Could you check a few things on this model? Use its own coordinates, in mm. A direction names the side the tool comes from. Coordinates: 2 decimals unless noted, no trailing zeros. Order: outer loops, then holes, each group sorted by start corner. A loop starts at its lowest first (then second) coordinate and runs counter-clockwise, first axis right, second up. Notation, with made-up numbers: (83, 18.25) -> (109, 18.25) arc R25 cw to (109, 47.25) -> close; hole circle Ø10 at (73.25, 80). An arc over 180 degrees is marked (long way). Use a Markdown table: item, result. Add a question column.
1) Thinking about a two-plate mould opening in Z: for faces 1 (the flat face through (19, 13, 5.802)), 2 (the flat face through (16.393, 29.272, -7.317)), 3 (the flat face through (17.3, 23.7, -7.1)), which applies, +Z half, -Z half, draft (parallel to the pull), parting line (faces both ways), or undercut?
2) If we section it at C-C (z = 4): Write out the boundary of the cut face in (x, y).
3) If I drill on L1, parallel to Z at x = 12.5, y = 17; L2, parallel to Y at x = 9.5, z = -11.25; L3, parallel to X at y = 15.25, z = -8, over which ranges is the centre line in solid material (lowest first)? Write a range as [from, to].
4) Will these pins go through, and if not, where does the flat tip stop? pin 1 Ø8 at (x, z) = (8, -13) entering from +Y; pin 2 Ø6 at (x, y) = (13.5, 20.5) entering from +Z; pin 3 Ø8 at (y, z) = (21, -3) entering from +X.
5) If we section it at B-B (x = 38): Write out the boundary of the cut face in (y, z).
6) Which directions (+Z, -Z, +X, -X, +Y, -Y) give clear straight access to the entire face, cutting with the end or side of a thin tool? Please do faces 4 (the flat face through (15, 21, -15.698)), 5 (the flat face through (18, 14, -2.957)), 6 (the flat face through (13, 18, -2.948)).
7) If we section it at A-A (z = -8.75): Write out the boundary of the cut face in (x, y), plus the area to 3 significant figures.
```python
from build123d import *

# Parameters (mm, degrees)
ESBO_O1_R                  = 1.5
RESSALTO_EXTRUS_O1_DEPTH   = 12
RESSALTO_EXTRUS_O1_2_DEPTH = 12
ESBO_O1_R_2                = 1.500000005
RESSALTO_EXTRUS_O1_3_DEPTH = 12
RESSALTO_EXTRUS_O1_4_DEPTH = 12
RESSALTO_EXTRUS_O1_5_DEPTH = 12
RESSALTO_EXTRUS_O1_6_DEPTH = 12
ESBO_O1_R_3                = 1.500000003
RESSALTO_EXTRUS_O1_7_DEPTH = 12
RESSALTO_EXTRUS_O1_8_DEPTH = 12
ESBO_O2_W                  = 79.998506149
ESBO_O2_H                  = 25.999999951
RESSALTO_EXTRUS_O2_DEPTH   = 3
ESBO_O3_W                  = 15
ESBO_O3_H                  = 17
RESSALTO_EXTRUS_O3_DEPTH   = 15
CHANFRO1_START             = 28.832866647
CHANFRO1_OUTLINE_W         = 17.320508076
CHANFRO1_OUTLINE_H         = 17
CHANFRO1_DEPTH             = 8.167133353
ESBO_O4_R                  = 7.5
CORTE_EXTRUS_O3_DEPTH      = 2
ESBO_O5_R                  = 3
CORTE_EXTRUS_O4_DEPTH      = 2
ESBO_O6_W                  = 8.5
ESBO_O6_H                  = 8.5
CORTE_EXTRUS_O5_DEPTH      = 9
ESBO_O7_W                  = 8.495190528
ESBO_O7_H                  = 8.490637191
CORTE_EXTRUS_O6_DEPTH      = 71.124048339
CORTE_EXTRUS_O7_START      = 1
ESBO_O10_W                 = 32.298347435
ESBO_O10_H                 = 12
CORTE_EXTRUS_O7_DEPTH      = 102
CORTE_EXTRUS_O9_REACH      = 63.707
ESBO_O13_W                 = 8.5
ESBO_O13_H                 = 3.123983639
ESBO_O14_W                 = 17
ESBO_O14_H                 = 3.169872981
CORTE_EXTRUS_O10_DEPTH     = 10


with BuildPart() as part:
    # Esbo_o1 → Ressalto-extrus_o1 (new body)
    with BuildSketch(Plane(origin=(0, 0, 0), x_dir=(1, 0, 0), z_dir=(0, 1, 0))):
        with Locations(Location((-18.866927397, -4.302093178, 0), (0, 0, 270))):
            Circle(ESBO_O1_R)
    extrude(amount=RESSALTO_EXTRUS_O1_DEPTH)



with BuildPart() as body_2:
    # Esbo_o1 → Ressalto-extrus_o1 2 (new body)
    with BuildSketch(Plane(origin=(0, 0, 0), x_dir=(1, 0, 0), z_dir=(0, 1, 0))):
        with Locations(Location((-18.868421246, 18.697906773, 0), (0, 0, 270))):
            Circle(ESBO_O1_R)
    extrude(amount=RESSALTO_EXTRUS_O1_2_DEPTH)


with BuildPart() as body_3:
    # Esbo_o1 → Ressalto-extrus_o1 3 (new body)
    with BuildSketch(Plane(origin=(0, 0, 0), x_dir=(1, 0, 0), z_dir=(0, 1, 0))):
        with Locations(Location((3.131578748, 18.697379942, 0), (0, 0, 270))):
            Circle(ESBO_O1_R_2)
    extrude(amount=RESSALTO_EXTRUS_O1_3_DEPTH)


with BuildPart() as body_4:
    # Esbo_o1 → Ressalto-extrus_o1 4 (new body)
    with BuildSketch(Plane(origin=(0, 0, 0), x_dir=(1, 0, 0), z_dir=(0, 1, 0))):
        with Locations(Location((3.133072603, -4.302620009, 0), (0, 0, 270))):
            Circle(ESBO_O1_R)
    extrude(amount=RESSALTO_EXTRUS_O1_4_DEPTH)


with BuildPart() as body_5:
    # Esbo_o1 → Ressalto-extrus_o1 5 (new body)
    with BuildSketch(Plane(origin=(0, 0, 0), x_dir=(1, 0, 0), z_dir=(0, 1, 0))):
        with Locations(Location((58.131578752, 18.697406939, 0), (0, 0, 270))):
            Circle(ESBO_O1_R)
    extrude(amount=RESSALTO_EXTRUS_O1_5_DEPTH)


with BuildPart() as body_6:
    # Esbo_o1 → Ressalto-extrus_o1 6 (new body)
    with BuildSketch(Plane(origin=(0, 0, 0), x_dir=(1, 0, 0), z_dir=(0, 1, 0))):
        with Locations(Location((58.131578752, -4.302593061, 0), (0, 0, 270))):
            Circle(ESBO_O1_R)
    extrude(amount=RESSALTO_EXTRUS_O1_6_DEPTH)


with BuildPart() as body_7:
    # Esbo_o1 → Ressalto-extrus_o1 7 (new body)
    with BuildSketch(Plane(origin=(0, 0, 0), x_dir=(1, 0, 0), z_dir=(0, 1, 0))):
        with Locations(Location((26.131578746, 18.696829164, 0), (0, 0, 270))):
            Circle(ESBO_O1_R_3)
    extrude(amount=RESSALTO_EXTRUS_O1_7_DEPTH)


with BuildPart() as body_8:
    # Esbo_o1 → Ressalto-extrus_o1 8 (new body)
    with BuildSketch(Plane(origin=(0, 0, 0), x_dir=(1, 0, 0), z_dir=(0, 1, 0))):
        with Locations(Location((26.133072603, -4.303170787, 0), (0, 0, 270))):
            Circle(ESBO_O1_R)
    extrude(amount=RESSALTO_EXTRUS_O1_8_DEPTH)


with BuildPart() as part_1:
    add(part.part)

    add(body_2.part)  # Ressalto-extrus_o2 merges body 2

    add(body_3.part)  # Ressalto-extrus_o2 merges body 3

    add(body_4.part)  # Ressalto-extrus_o2 merges body 4

    add(body_5.part)  # Ressalto-extrus_o2 merges body 5

    add(body_6.part)  # Ressalto-extrus_o2 merges body 6

    add(body_7.part)  # Ressalto-extrus_o2 merges body 7

    add(body_8.part)  # Ressalto-extrus_o2 merges body 8
    # Esbo_o2 → Ressalto-extrus_o2 (add)
    with BuildSketch(Plane(origin=(0, 12, 0), x_dir=(1, 0, 0), z_dir=(0, 1, 0))):
        with Locations((19.632325677, 7.197906797)):
            Rectangle(ESBO_O2_W, ESBO_O2_H)
    extrude(amount=RESSALTO_EXTRUS_O2_DEPTH)

    # Esbo_o3 → Ressalto-extrus_o3 (add)
    with BuildSketch(Plane(origin=(0, 15, 0), x_dir=(1, 0, 0), z_dir=(0, 1, 0))):
        with Locations((17.133072603, 7.197906773)):
            Rectangle(ESBO_O3_W, ESBO_O3_H)
    extrude(amount=RESSALTO_EXTRUS_O3_DEPTH)

    # Chanfro1: read off the stored shape, not the designer's step
    # Chanfro1 outline → Chanfro1 (cut)
    with BuildSketch(Plane(origin=(0, 0, 0), x_dir=(0.49999999999999767, -0.86602540378444, 0), z_dir=(0.8660254037844399, 0.49999999999999795, 0)).offset(CHANFRO1_START)):
        with Locations((-9.334098793, 7.197906773)):
            Rectangle(CHANFRO1_OUTLINE_W, CHANFRO1_OUTLINE_H)
    extrude(amount=CHANFRO1_DEPTH, mode=Mode.SUBTRACT)

    # Esbo_o4 → Corte-extrus_o3 (cut)
    with BuildSketch(Plane(origin=(24.96999498, 14.416433324, 0), x_dir=(0, 0, -1), z_dir=(0.8660254037844396, 0.4999999999999982, 0))):
        with Locations(Location((7.197906773, 8.673844755, 0), (0, 0, 90))):
            Circle(ESBO_O4_R)
    extrude(amount=-CORTE_EXTRUS_O3_DEPTH, mode=Mode.SUBTRACT)

    # Esbo_o5 → Corte-extrus_o4 (cut)
    with BuildSketch(Plane(origin=(23.237944173, 13.416433324, 0), x_dir=(0, 0, -1), z_dir=(0.8660254037844398, 0.4999999999999983, 0))):
        with Locations(Location((7.197906773, 8.673844755, 0), (0, 0, 90))):
            Circle(ESBO_O5_R)
    extrude(amount=-CORTE_EXTRUS_O4_DEPTH, mode=Mode.SUBTRACT)

    # Esbo_o6 → Corte-extrus_o5 (cut)
    with BuildSketch(Plane(origin=(21.505893365, 12.416433324, 0), x_dir=(0, 0, -1), z_dir=(0.8660254037844396, 0.49999999999999833, 0))):
        with Locations((7.197906773, 8.673844755)):
            Rectangle(ESBO_O6_W, ESBO_O6_H)
    extrude(amount=-CORTE_EXTRUS_O5_DEPTH, mode=Mode.SUBTRACT)

    # Esbo_o7 → Corte-extrus_o6 (cut, through all)
    with BuildSketch(Plane(origin=(-2.211922378, 3.831161941, 0), x_dir=(0.8660254037844396, 0.49999999999999845, 0), z_dir=(-0.49999999999999845, 0.8660254037844396, 0))):
        with Locations((20.585271383, 7.202588178)):
            Rectangle(ESBO_O7_W, ESBO_O7_H)
    extrude(amount=-CORTE_EXTRUS_O6_DEPTH, mode=Mode.SUBTRACT)

    # Esbo_o10 → Corte-extrus_o7 (cut)
    with BuildSketch(Plane.ZY.offset(20.366927397).offset(CORTE_EXTRUS_O7_START)):
        with Locations((-7.642594808, 6)):
            Rectangle(ESBO_O10_W, ESBO_O10_H)
    extrude(amount=-CORTE_EXTRUS_O7_DEPTH, mode=Mode.SUBTRACT)

    # Corte-extrus_o9: up to this plane
    corte_extrus_o9_end = Plane(origin=(21.505893365, 12.416433324, 0), z_dir=(0.8660254037844397, 0.49999999999999806, 0))
    # Esbo_o13 → Corte-extrus_o9 (cut, up to the surface)
    with BuildSketch(Plane.ZY.offset(-9.633072603), mode=Mode.PRIVATE) as corte_extrus_o9_sk1:
        with Locations((-7.197906773, 22.046819377)):
            Rectangle(ESBO_O13_W, ESBO_O13_H)
    corte_extrus_o9_tool1 = split(extrude(corte_extrus_o9_sk1.sketch, amount=-CORTE_EXTRUS_O9_REACH, mode=Mode.PRIVATE), bisect_by=corte_extrus_o9_end, keep=Keep.BOTH, mode=Mode.PRIVATE)
    add(corte_extrus_o9_tool1.solids().sort_by_distance((9.633073, 22.046819, -7.197907))[0], mode=Mode.SUBTRACT)

    # Esbo_o14 → Corte-extrus_o10 (cut)
    with BuildSketch(Plane(origin=(24.96999498, 14.416433324, 0), x_dir=(0, 0, -1), z_dir=(0.8660254037844396, 0.4999999999999985, 0))):
        with Locations((7.197906773, 19.579289321)):
            Rectangle(ESBO_O14_W, ESBO_O14_H)
    extrude(amount=-CORTE_EXTRUS_O10_DEPTH, mode=Mode.SUBTRACT)


solid = part_1.part
```
Answer sheet:
| question | item | result |
|---|---|---|
| 1 | face 1 | +Z half |
| 1 | face 2 | draft |
| 1 | face 3 | undercut |
| 2 | outline | (-20.37, 12) -> (59.63, 12) -> (59.63, 15) -> (-20.37, 15) -> close |
| 3 | L1 | [-15.7, -11.45], [-2.95, 1.3] |
| 3 | L2 | [12, 15] |
| 3 | L3 | [19.87, 22.18], [23.98, 24.49] |
| 4 | pin 1 | y = 27.71 |
| 4 | pin 2 | z = 1.3 |
| 4 | pin 3 | x = 23.43 |
| 5 | outline | (12, -20.2) -> (15, -20.2) -> (15, 5.8) -> (12, 5.8) -> close |
| 6 | face 4 | -Z, +X, -X, +Y |
| 6 | face 5 | -Y |
| 6 | face 6 | none |
| 7 | outline | (-20.37, 12) -> (11.35, 12) -> (9.62, 15) -> (-20.37, 15) -> close; (9.63, 23.61) -> (15.04, 23.61) -> (15.89, 22.15) -> (17.62, 23.15) -> (15.23, 27.28) -> (16.96, 28.28) -> (15.97, 30) -> (9.63, 26.34) -> close; (18.45, 17.7) -> (21.75, 12) -> (59.63, 12) -> (59.63, 15) -> (24.63, 15) -> (24.3, 15.57) -> (22.57, 14.57) -> (20.18, 18.7) -> close |
| 7 | area | 250 mm2 |
